Part print with two shaded views. Sizes in mm from the minimum x, y, z corner. Round coordinates to 2 decimals unless told otherwise and drop trailing zeros. Loops run counter-clockwise (first coordinate to the right, second up) from the corner with the lowest first, then second, coordinate; pieces in that order, holes last. Notation, with made-up numbers: (55, 31) -> (84, 31) arc R18 ccw to (84, 44) -> close; hole circle Ø9 at (65, 80.5). An arc over 180 degrees is marked (long way). Use a Markdown table: item, result. Add a question column.
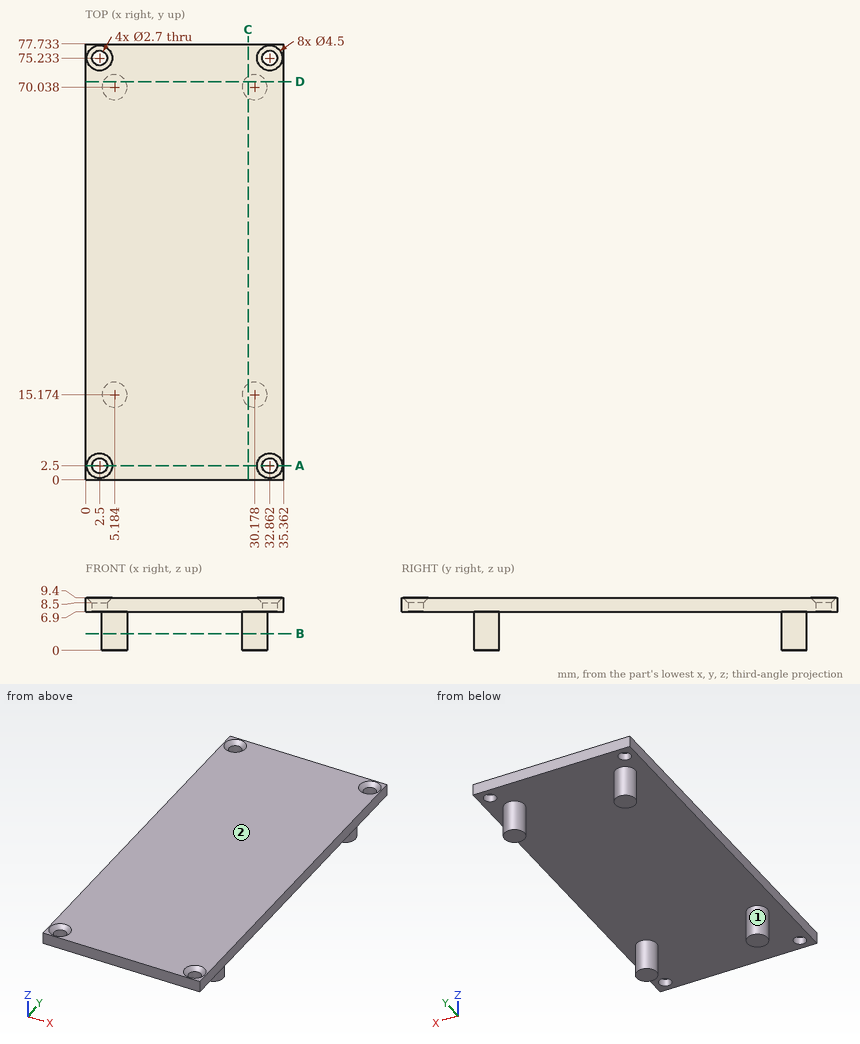
1) Cut at D-D on y = 71. Write the cut outline in (x, z).
2) Cut at B-B on z = 3. Count the separate pieces of the cut face and the enclosed holes in it.
3) Pin check, flat tip, straight feed: pin 1 Ø3 at (x, y) = (32.86, 75.23) entering from -Z. Stop position of the tip, or through.
4) Cut at C-C on x = 29. Write the cut outline in (y, z) (1 decimal), and give its area (3 significant figures).
5) Cut at A-A on y = 2.5. Write the cut outline in (x, z).
6) Wall check: probe 1 along Y at (x, z) = (2.5, 7.2); probe 2 along Z at (x, y) = (26.5, 52.5); probe 3 along X at (y, z) = (69.5, 5.75). Give the ranges that are in metal, low to high. Write a range as from..to.
7) Pull direction X, two halves, no side cores. Call the marked faces 1 and 2: +X half, -X half, draft (parallel to the pull), parting line (faces both ways), or undercut.
Established:
| question | item | result |
|---|---|---|
| 1 | outline | (0, 6.9) -> (3.15, 6.9) -> (3.15, 0) -> (7.22, 0) -> (7.22, 6.9) -> (28.14, 6.9) -> (28.14, 0) -> (32.21, 0) -> (32.21, 6.9) -> (35.36, 6.9) -> (35.36, 9.4) -> (0, 9.4) -> close |
| 2 | separate pieces | 4 |
| 2 | enclosed holes | 0 |
| 3 | pin 1 | stops at z = 6.9 |
| 4 | outline | (0, 6.9) -> (13.3, 6.9) -> (13.3, 0) -> (17.1, 0) -> (17.1, 6.9) -> (68.1, 6.9) -> (68.1, 0) -> (72, 0) -> (72, 6.9) -> (77.7, 6.9) -> (77.7, 9.4) -> (0, 9.4) -> close |
| 4 | area | 247 mm^2 |
| 5 | outline | (0, 6.9) -> (1.15, 6.9) -> (1.15, 8.5) -> (0.25, 9.4) -> (0, 9.4) -> close; (3.85, 6.9) -> (31.51, 6.9) -> (31.51, 8.5) -> (30.61, 9.4) -> (4.75, 9.4) -> (3.85, 8.5) -> close; (34.21, 6.9) -> (35.36, 6.9) -> (35.36, 9.4) -> (35.11, 9.4) -> (34.21, 8.5) -> close |
| 6 | probe 1 | y = 0..1.15, 3.85..73.88, 76.58..77.73 |
| 6 | probe 2 | z = 6.9..9.4 |
| 6 | probe 3 | x = 3..7.37, 27.99..32.36 |
| 7 | face 1 | undercut |
| 7 | face 2 | draft |
